The listing builds one solid part. Answer for the finished solid, in the listing's coordinates (mm). A direction names the side the tool comes from. Give positions to 0.01 mm unless a question says otherwise; leave off trailing zeros. Loops run counter-clockwise (first coordinate to the right, second up) from the corner with the lowest first, then second, coordinate; pieces in that order, holes last. Notation, with made-up numbers: (34.5, 47.25) -> (38.5, 47.25) arc R33 cw to (38.5, 78.25) -> close; hole circle Ø4 at (-18, -23.75). An arc over 180 degrees is marked (long way). One line per question, with ' | ' between items. Start each with the question number.
from build123d import *

# Parameters (mm, degrees)
SKETCH1_W           = 24
SKETCH1_H           = 24
BOSS_EXTRUDE1_DEPTH = 20
SKETCH2_W           = 8
SKETCH2_H           = 24
BOSS_EXTRUDE2_DEPTH = 25.4
SKETCH3_R           = 1.65
CUT_EXTRUDE1_DEPTH  = 15


with BuildPart() as part:
    # Sketch1 → Boss-Extrude1 (new body)
    with BuildSketch(Plane(origin=(0, 0, 0), x_dir=(1, 0, 0), z_dir=(0, 1, 0))):
        with Locations((12, 12)):
            Rectangle(SKETCH1_W, SKETCH1_H)
    extrude(amount=BOSS_EXTRUDE1_DEPTH)

    # Sketch2 → Boss-Extrude2 (add)
    with BuildSketch(Plane(origin=(0, 20, 0), x_dir=(1, 0, 0), z_dir=(0, 1, 0))):
        with Locations((20, 12)):
            Rectangle(SKETCH2_W, SKETCH2_H)
    extrude(amount=BOSS_EXTRUDE2_DEPTH)

    # Sketch3 → Cut-Extrude1 (cut)
    with BuildSketch(Plane(origin=(0, 0, 0), x_dir=(-1, 0, 0), z_dir=(0, -1, 0))):
        with Locations(Location((-4, 16, 0), (0, 0, 90))):
            Circle(SKETCH3_R)
        with Locations(Location((-4, 8, 0), (0, 0, 90))):
            Circle(SKETCH3_R)
        with Locations(Location((-12, 8, 0), (0, 0, 90))):
            Circle(SKETCH3_R)
        with Locations(Location((-12, 16, 0), (0, 0, 90))):
            Circle(SKETCH3_R)
        with Locations(Location((-20, 8, 0), (0, 0, 90))):
            Circle(SKETCH3_R)
        with Locations(Location((-20, 16, 0), (0, 0, 90))):
            Circle(SKETCH3_R)
    extrude(amount=-CUT_EXTRUDE1_DEPTH, mode=Mode.SUBTRACT)


solid = part.part
1. The part is cut by section C-C (x = 12). Write down the section's boundary in (y, z), plus the area to 3 significant figures.
2. Straight lines are drawn through the part: L1, parallel to X at y = 10.75, z = -16; L2, parallel to Z at x = 13.5, y = 3.5; L3, parallel to X at y = 24.5, z = -1.75. For each, find the intervals that lie inside material, in ascending order.
3. Determine the mould class of faces 1 (the cylindrical face through (10.4, 7.4, -7.6)), 2 (the flat face through (16, 33, -12)), 3 (the flat face through (14, 17, 0)) for opening direction Z: released by +Z, released by -Z, zero draft, split by the parting line, or undercut.
4. The part is cut by section A-A (y = 10.5). Write down the section's boundary in (x, z).
5. The part is cut by section B-B (z = -8). Write down the section's boundary in (x, y).
6. For faces 4 (the cylindrical face through (21.636, 7.395, -7.785)), 5 (the flat face through (0, 10, -12)), 6 (the flat face through (8, 20, -12)), determine the directions among +Z, -Z, +X, -X, +Y, -Y from which every point of the face is accessible in a straight line to the end or side of a thin tool.
7. Each of these flat-tipped pins is pushed along its axis until it touches: pin 1 Ø3 at (x, z) = (12, -8) entering from -Y; pin 2 Ø1.5 at (y, z) = (36.5, -3.5) entering from -X; pin 3 Ø3 at (x, z) = (4, -16) entering from +Y; pin 4 Ø12 at (x, y) = (14.5, 17.5) entering from +Z. Where does it stop, or does it pass through?
8. The part is cut by section D-D (z = -20). Write down the section's boundary in (x, y).
Check sheet entries:
1) outline: (0, -24) -> (20, -24) -> (20, 0) -> (0, 0) -> (0, -6.35) -> (15, -6.35) -> (15, -9.65) -> (0, -9.65) -> (0, -14.35) -> (15, -14.35) -> (15, -17.65) -> (0, -17.65) -> close | area: 381 mm^2
2) L1: x = 0 to 2.35, 5.65 to 10.35, 13.65 to 18.35, 21.65 to 24 | L2: z = -24 to -16.69, -15.31 to -8.69, -7.31 to 0 | L3: x = 16 to 24
3) face 1: undercut | face 2: zero draft | face 3: released by +Z
4) outline: (0, -24) -> (24, -24) -> (24, 0) -> (0, 0) -> close; hole circle Ø3.3 at (4, -16); hole circle Ø3.3 at (4, -8); hole circle Ø3.3 at (12, -16); hole circle Ø3.3 at (12, -8); hole circle Ø3.3 at (20, -16); hole circle Ø3.3 at (20, -8)
5) outline: (0, 0) -> (2.35, 0) -> (2.35, 15) -> (5.65, 15) -> (5.65, 0) -> (10.35, 0) -> (10.35, 15) -> (13.65, 15) -> (13.65, 0) -> (18.35, 0) -> (18.35, 15) -> (21.65, 15) -> (21.65, 0) -> (24, 0) -> (24, 45.4) -> (16, 45.4) -> (16, 20) -> (0, 20) -> close
6) face 4: -Y | face 5: +Z, -Z, -X, +Y, -Y | face 6: +Z, -Z, -X, +Y
7) pin 1: stops at y = 15 | pin 2: stops at x = 16 | pin 3: stops at y = 20 | pin 4: stops at z = 0
8) outline: (0, 0) -> (24, 0) -> (24, 45.4) -> (16, 45.4) -> (16, 20) -> (0, 20) -> close
